Autodesk Inventor part; units mm, degrees
ref_plane "YZ Plane" through (0, 0, 0) normal (1, 0, 0) x (0, 1, 0)
ref_plane "XZ Plane" through (0, 0, 0) normal (0, 1, 0) x (-1, 0, 0)
ref_plane "XY Plane" through (0, 0, 0) normal (0, 0, 1) x (1, 0, 0)
sketch "스케치1" plane through (0, 0, 0) normal (0, 0, 1) x (1, 0, 0)
  line L0 (-25, 55) -> (25, 55)
  line L1 (25, 55) -> (25, -55)
  line L2 (25, -55) -> (-25, -55)
  line L3 (-25, -55) -> (-25, 55)
  line L4 (-25, 55) -> (25, -55) construction
  line L5 (25, 55) -> (-25, -55) construction
  point P0 (0, 0)
  dimension "d0" = 50
  dimension "d1" = 110
extrude "돌출1" add sketch "스케치1" along normal blind 41.5
sketch "스케치2" plane through (-25, -55, 0) normal (0, -1, 0) x (1, 0, 0)
  line L0 (50, 0) -> (0, 0)
  line L1 (0, 0) -> (25, 0)
  line L2 (25, 0) -> (25, 41.5)
  line L3 (50, 41.5) -> (0, 41.5)
  circle A0 centre (25, 41.5) radius 21.2
  dimension "d4" = 42.4
extrude "돌출2" cut sketch "스케치2" against normal blind 51.9
sketch "스케치3" plane through (-25, -3.1, 0) normal (0, -1, 0) x (1, 0, 0)
  line L0 (0, 0) -> (25, 0)
  line L1 (0, 0) -> (50, 0)
  line L2 (25, 0) -> (25, 41.5)
  line L3 (50, 41.5) -> (0, 41.5)
  circle A0 centre (25, 41.5) radius 22.3
  dimension "d7" = 44.6
extrude "돌출3" cut sketch "스케치3" against normal blind 30
sketch "스케치4" plane through (-25, 26.9, 0) normal (0, -1, 0) x (1, 0, 0)
  line L0 (50, 0) -> (0, 0)
  line L1 (0, 0) -> (25, 0)
  line L2 (25, 0) -> (25, 41.5)
  line L3 (50, 41.5) -> (0, 41.5)
  circle A0 centre (25, 41.5) radius 21.2
  dimension "d10" = 42.4
extrude "돌출4" cut sketch "스케치4" against normal through all
fillet "모깎기1" radius 2 2 edges at (-25, 0, 41.5) (25, 0, 41.5)
sketch "스케치5" plane through (-25, 55, 0) normal (0, 1, 0) x (1, 0, 0)
  arc A0 (47.3, -41.5) -> (2.7, -41.5) centre (25, -41.5) ccw
  arc A1 (47.3, -41.5) -> (2.7, -41.5) centre (25, -41.5) ccw
  line L0 (0, 0) -> (0, -39.5)
  line L1 (50, 0) -> (50, -39.5)
  line L2 (0, 0) -> (50, 0)
  line L3 (50, 0) -> (50, -19)
  line L4 (50, -19) -> (0, -19)
  line L5 (0, -19) -> (0, 0)
  point P0 (25, 0)
  dimension "d15" = 19
extrude "돌출5" cut sketch "스케치5" against normal through all
properties part number "motor_support2" material "ABS 플라스틱"
Check sheet for the modelled part. Datum: model origin and axes. Units: mm. A direction names the side the tool comes from. Round coordinates to 2 decimals unless told otherwise and drop trailing zeros. Order: outer loops, then holes, each group sorted by start corner. A loop starts at its lowest first (then second) coordinate and runs counter-clockwise, first axis right, second up.
1) Mould release check, pull along Y, two halves, no side actions. Record for faces 1 (the flat face through (3, -3.1, 20)), 2 (the flat face through (0, -55, 20)), 3 (the flat face through (3, 26.9, 20)), 4 (the cylindrical face through (-0.466, -29.413, 20.305)): +Y half, -Y half, draft (parallel to the pull), parting line (faces both ways), or undercut.
2) Section check A-A (z = 24). Record the boundary of the cut face in (x, y).
3) Section check C-C (x = 0). Record the boundary of the cut face in (y, z), and give its area (3 significant figures).
4) Tool access check on faces 5 (the cylindrical face through (-0.49, 11.69, 19.205)), 6 (the cylindrical face through (24.43, -0.77, 40.9)). Record the directions out of +Z, -Z, +X, -X, +Y, -Y that give a thin tool (end or side, any length) a straight path to the whole face; none if there is none.
5) Section check B-B (y = 9). Record the boundary of the cut face in (x, z).
6) Section check D-D (z = 35). Record the boundary of the cut face in (x, y).
7) Go/stop test with flat-tipped pins: pin 1 Ø8 at (x, z) = (-18, 36) entering from -Y; pin 2 Ø6.5 at (x, z) = (9, 29) entering from +Y; pin 3 Ø12 at (x, y) = (-8, -29.5) entering from +Z. Record where each tip stops, or that it passes through.
8) Scan lines: line 1 (Z direction, x = 1, y = -22); line 2 (X direction, y = -25.5, z = 22.75); line 3 (X direction, y = 13.5, z = 38). Record each from-to range of solid material in increasing order.
Result:
1. face 1: undercut
1. face 2: -Y half
1. face 3: undercut
1. face 4: draft
2. outline: (-25, -55) - (-11.97, -55) - (-11.97, -3.1) - (-13.82, -3.1) - (-13.82, 26.9) - (-11.97, 26.9) - (-11.97, 55) - (-25, 55) - close; (11.97, -55) - (25, -55) - (25, 55) - (11.97, 55) - (11.97, 26.9) - (13.82, 26.9) - (13.82, -3.1) - (11.97, -3.1) - close
3. outline: (-55, 19) - (55, 19) - (55, 20.3) - (26.9, 20.3) - (26.9, 19.2) - (-3.1, 19.2) - (-3.1, 20.3) - (-55, 20.3) - close
3. area: 110 mm2
4. face 5: +Z
4. face 6: +Z, +X, +Y, -Y
5. outline: (-25, 19) - (25, 19) - (25, 39.5) arc R2 ccw to (23, 41.5) - (22.3, 41.5) arc R22.3 cw to (-22.3, 41.5) - (-23, 41.5) arc R2 ccw to (-25, 39.5) - close
6. outline: (-25, -55) - (-20.18, -55) - (-20.18, -3.1) - (-21.33, -3.1) - (-21.33, 26.9) - (-20.18, 26.9) - (-20.18, 55) - (-25, 55) - close; (20.18, -55) - (25, -55) - (25, 55) - (20.18, 55) - (20.18, 26.9) - (21.33, 26.9) - (21.33, -3.1) - (20.18, -3.1) - close
7. pin 1: stops at y = -55
7. pin 2: passes through
7. pin 3: stops at z = 25.58
8. line 1: z = 19 to 20.32
8. line 2: x = -25 to -9.89, 9.89 to 25
8. line 3: x = -25 to -22.02, 22.02 to 25
